Read the model definition and answer for the solid it produces. Units are mm, in the model's axes. A direction names the side the tool comes from. Coordinates: 2 decimals unless noted, no trailing zeros. Order: outer loops, then holes, each group sorted by start corner. A loop starts at its lowest first (then second) coordinate and runs counter-clockwise, first axis right, second up. Notation, with made-up numbers: M -14.5,29.25 L 37.5,29.25 A7 cw 37.5,41.25 Z; hole C -10,85 d7. An arc over 180 degrees is marked long. Put each result on its own line as item: value.
from build123d import *

# Parameters (mm, degrees)
ESQUISSE1_W             = 20
ESQUISSE1_H             = 10
BOSS_EXTRU_1_DEPTH      = 5
BOSS_EXTRU_1_DEPTH_BACK = 5
ESQUISSE3_R             = 2.5
ENL_V_MAT_EXTRU_1_DEPTH = 26


with BuildPart() as part:
    # Esquisse1 → Boss.-Extru.1 (new body, two sides)
    with BuildSketch(Plane.XY) as boss_extru_1_sk:
        Polygon((-20, 15), (20, 15), (20, -10), (5, -10), (5, -30), (2, -30), (2, -20), (-2, -20), (-2, -30), (-5, -30), (-5, -10), (-20, -10), align=None)
        Rectangle(ESQUISSE1_W, ESQUISSE1_H, mode=Mode.SUBTRACT)
    extrude(amount=BOSS_EXTRU_1_DEPTH)
    extrude(boss_extru_1_sk.sketch, amount=-BOSS_EXTRU_1_DEPTH_BACK)

    # Esquisse3 → Enl_v. mat.-Extru.1 (cut, through all)
    with BuildSketch(Plane(origin=(5, 0, 0), x_dir=(0, 0, -1), z_dir=(1, 0, 0))):
        with Locations((0, -25)):
            Circle(ESQUISSE3_R)
    extrude(amount=-ENL_V_MAT_EXTRU_1_DEPTH, mode=Mode.SUBTRACT)


solid = part.part
Q1. A tool of negligible diameter and unlimited length cuts with its end or side. For faces 4 (the face through (-12, -10, 0)), 5 (the face through (2, -27, 2)), 6 (the face through (0, 5, 0)), from which of +Z, -Z, +X, -X, +Y, -Y can it reach the whole face along a straight path? Write none if from no direction.
Answers below:
face 4: +Z, -Z, -X, -Y
face 5: +Z, -Z, -Y
face 6: +Z, -Z
Q2. Consider line 1 along Y through (x, z) = (-3.35, 0); line 2 along X through (y, z) = (1.5, -2.75); line 3 along X through (y, z) = (-23.5, -3.75). Determine where each line is inside the solid, lowest interval first.
Answers below:
line 1: y = -30 to -27.5, -22.5 to -5, 5 to 15
line 2: x = -20 to -10, 10 to 20
line 3: x = -5 to -2, 2 to 5
Q3. For a pull along Y with two mould halves and no side action, classify faces 1 (the face through (0, 15, 0)), 2 (the face through (-10, 0, 0)), 3 (the face through (0, -7, -5)) as +Y half, -Y half, draft (parallel to the pull), parting line (faces both ways), or undercut.
Answers below:
face 1: +Y half
face 2: undercut
face 3: draft
Q4. Find section A-A on z = 0. Write down the section's boundary in (x, y).
Answers below:
outline: M -20,-10 L -5,-10 L -5,-22.5 L -2,-22.5 L -2,-20 L 2,-20 L 2,-22.5 L 5,-22.5 L 5,-10 L 20,-10 L 20,15 L -20,15 Z; M -5,-30 L -2,-30 L -2,-27.5 L -5,-27.5 Z; M 2,-30 L 5,-30 L 5,-27.5 L 2,-27.5 Z; hole M -10,-5 L 10,-5 L 10,5 L -10,5 Z
Q5. Find section B-B on y = -22. Write down the section's boundary in (x, z).
Answers below:
outline: M -5,-5 L -2,-5 L -2,5 L -5,5 Z; M 2,-5 L 5,-5 L 5,5 L 2,5 Z
Q6. Find section C-C on x = -4. Write down the section's boundary in (y, z).
Answers below:
outline: M -30,-5 L -5,-5 L -5,5 L -30,5 Z; M 5,-5 L 15,-5 L 15,5 L 5,5 Z; hole C -25,0 d5
Q7. Given pin 1 (3 mm diameter, centred on x = 15, z = 0, fed in from -Y); pin 2 (6 mm diameter, centred on y = -25, z = 0, fed in from +X), each flat-ended and moving along its own axis, determine where each tip first touches the part or whether it passes through.
Answers below:
pin 1: stops at y = -10
pin 2: stops at x = 5
Q8. Find section D-D on z = 3.5. Write down the section's boundary in (x, y), plus the area to 3 significant figures.
Answers below:
outline: M -20,-10 L -5,-10 L -5,-30 L -2,-30 L -2,-20 L 2,-20 L 2,-30 L 5,-30 L 5,-10 L 20,-10 L 20,15 L -20,15 Z; hole M -10,-5 L 10,-5 L 10,5 L -10,5 Z
area: 960 mm^2
